The model under review builds one solid part; all positions refer to its coordinate system, in mm. A direction names the side the tool comes from. Give positions to 0.01 mm unless a question says otherwise; leave off trailing zeros. Order: outer loops, then holes, each group sorted by start corner. A loop starts at its lowest first (then second) coordinate and runs counter-clockwise, first axis right, second up. Notation, with made-up numbers: (35, 11) - (59, 11) arc R31 ccw to (59, 40) - close; hole circle Ø10 at (34.25, 47). An arc over 180 degrees is marked (long way). Use CSV: the item, a comma, the result in double quotes.
```python
from build123d import *

# Parameters (mm, degrees)
MB_DEPTH    = 40.5
CAM_DEPTH   = 40.5
LENTE_DEPTH = 8


with BuildPart() as part:
    # Croquis_mb → MB (new body)
    with BuildSketch(Plane.XY.offset(-128.1)):
        Polygon((-123.543957493, 167.071730093), (-106.238601826, 187.796706939), (-105.01045505, 186.771204381), (-122.315810717, 166.046227535), align=None)
    extrude(amount=MB_DEPTH)

    # Croquis_cam → CAM (add)
    with BuildSketch(Plane.XY.offset(-128.1)):
        Polygon((-121.835106393, 166.621921336), (-105.491159374, 186.195510579), (-97.201168636, 179.273368313), (-113.545115654, 159.69977907), align=None)
    extrude(amount=CAM_DEPTH)

    # Croquis_lente → Lente (add)
    with BuildSketch(Plane.XY.offset(-103.85)):
        Polygon((-107.93689854, 166.416206751), (-102.80938575, 172.556940631), (-97.436243605, 168.07036694), (-102.563756395, 161.92963306), align=None)
    extrude(amount=-LENTE_DEPTH)


solid = part.part
```
Item 1: Wall thickness on L1, parallel to X at y = 172, z = -96; L2, parallel to X at y = 173, z = -124.5; L3, parallel to Y at x = -99.75, z = -122: over which ranges is each line inside the solid? List them lowest first.
Results list:
L1,"x = -119.43 to -103.27"
L2,"x = -118.59 to -102.44"
L3,"y = 176.22 to 181.4"
Item 2: Tool access review of faces 4 (the face through (-103, 167, -111.85)), 5 (the face through (-103, 167, -103.85)), 6 (the face through (-100, 165, -108)): name each direction out of +Z, -Z, +X, -X, +Y, -Y from which nothing blocks a thin tool from reaching the whole face with its end or side.
Results list:
face 4,"-Z, +X, -Y"
face 5,"+Z, +X, -Y"
face 6,"+Z, -Z, +X, -Y"
Item 3: Take a section at C-C, the plane y = 171.75. Give the boundary of the cut face in (x, z), and give its area (3 significant figures).
Results list:
outline,"(-119.64, -128.1) - (-103.48, -128.1) - (-103.48, -111.85) - (-101.84, -111.85) - (-101.84, -103.85) - (-103.48, -103.85) - (-103.48, -87.6) - (-119.64, -87.6) - close"
area,"667 mm2"
Item 4: Clearance check with flat-ended pins moving along their axes: pin 1 (4 mm diameter, centred on y = 169.5, z = -100.5, fed in from +X); pin 2 (2 mm diameter, centred on x = -109, z = -97, fed in from -Y); pin 3 (5 mm diameter, centred on y = 162.5, z = -99.5, fed in from +X); pin 4 (8.5 mm diameter, centred on x = -102.5, y = 167, fed in from -Z). State where each tip first meets the part, or that it passes through.
Results list:
pin 1,"stops at x = -103.69"
pin 2,"stops at y = 163.95"
pin 3,"stops at x = -109.12"
pin 4,"stops at z = -128.1"
Item 5: Take a section at B-B, the plane y = 164. Give the boundary of the cut face in (x, z) (3 decimals).
Results list:
outline,"(-118.695, -128.1) - (-109.954, -128.1) - (-109.954, -87.6) - (-118.695, -87.6) - close; (-105.043, -111.85) - (-100.835, -111.85) - (-100.835, -103.85) - (-105.043, -103.85) - close"
Item 6: Mouldability with a two-part tool opening along X and no side actions: class faces 1 (the face through (-100.16, 170.345, -107.794)), 2 (the face through (-105.21, 164.14, -107.79)), 3 (the face through (-122.92, 166.55, -108.13)) as pulls with the +X half, pulls with the -X half, needs draft (parallel to the pull), parting line crosses it, or undercut.
Results list:
face 1,"pulls with the +X half"
face 2,"undercut"
face 3,"pulls with the -X half"
Item 7: Take a section at D-D, the plane z = -109. Give the boundary of the cut face in (x, y).
Results list:
outline,"(-123.54, 167.07) - (-122.32, 166.05) - (-121.84, 166.62) - (-113.55, 159.7) - (-107.94, 166.42) - (-102.56, 161.93) - (-97.44, 168.07) - (-102.81, 172.56) - (-97.2, 179.27) - (-105.49, 186.2) - (-105.01, 186.77) - (-106.24, 187.8) - close"
Item 8: Take a section at A-A, the plane z = -114.5. Give the boundary of the cut face in (x, y), and give its area (3 significant figures).
Results list:
outline,"(-123.54, 167.07) - (-122.32, 166.05) - (-121.84, 166.62) - (-113.55, 159.7) - (-97.2, 179.27) - (-105.49, 186.2) - (-105.01, 186.77) - (-106.24, 187.8) - close"
area,"319 mm2"
